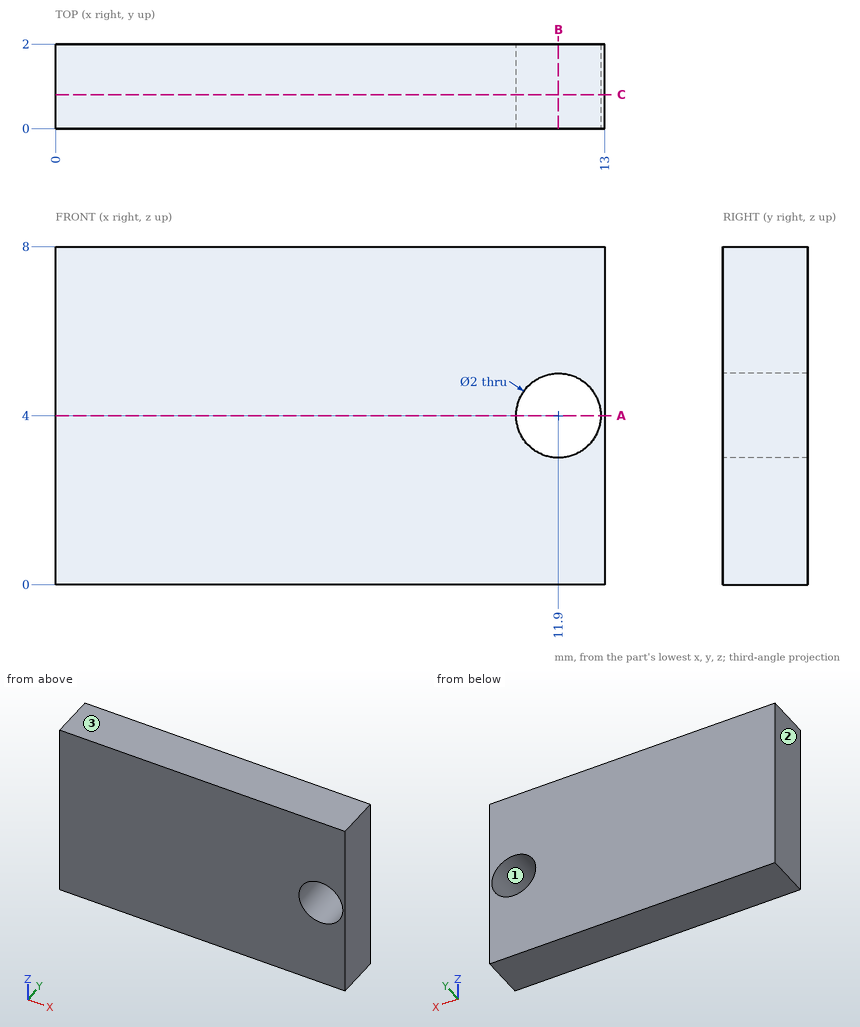
Study the drawing (mm; zero at the part's minimum x, y, z) and answer. Round coordinates to 2 decimals unless told otherwise and drop trailing zeros. Loops run counter-clockwise (first coordinate to the right, second up) from the corner with the lowest first, then second, coordinate; pieces in that order, holes last. Notation, with made-up numbers: (42.25, 52.5) -> (46.25, 52.5) arc R24 cw to (46.25, 67.5) -> close; hole circle Ø3 at (13.5, 52.25). An arc over 180 degrees is marked (long way). One line per item, written item: value.
1) A cutting plane is placed at C-C (y = 0.8). Determine the outline of the cut face in (x, z).
Answer list:
outline: (0, 0) -> (13, 0) -> (13, 8) -> (0, 8) -> close; hole circle Ø2 at (11.9, 4)
2) A cutting plane is placed at A-A (z = 4). Determine the outline of the cut face in (x, y), and give its area (3 significant figures).
Answer list:
outline: (0, 0) -> (10.9, 0) -> (10.9, 2) -> (0, 2) -> close; (12.9, 0) -> (13, 0) -> (13, 2) -> (12.9, 2) -> close
area: 22.0 mm²
3) The mould has two halves that part along X. Classify the marked faces 1, 2 and 3: pulls with the +X half, pulls with the -X half, needs draft (parallel to the pull), parting line crosses it, or undercut.
Answer list:
face 1: undercut
face 2: pulls with the -X half
face 3: needs draft
4) Consider L1, parallel to Z at x = 11.9, y = 0.7; L2, parallel to X at y = 0.4, z = 4.75; L3, parallel to X at y = 1, z = 4.5. Determine where each line is inside the solid, lowest interval first. Write a range as [from, to].
Answer list:
L1: z = [0, 3], [5, 8]
L2: x = [0, 11.24], [12.56, 13]
L3: x = [0, 11.03], [12.77, 13]
5) A cutting plane is placed at B-B (x = 11.9). Determine the outline of the cut face in (y, z).
Answer list:
outline: (0, 0) -> (2, 0) -> (2, 3) -> (0, 3) -> close; (0, 5) -> (2, 5) -> (2, 8) -> (0, 8) -> close
